Autodesk Inventor part; units mm, degrees
ref_plane "YZ Plane" through (0, 0, 0) normal (1, 0, 0) x (0, 1, 0)
ref_plane "XZ Plane" through (0, 0, 0) normal (0, 1, 0) x (-1, 0, 0)
ref_plane "XY Plane" through (0, 0, 0) normal (0, 0, 1) x (1, 0, 0)
sketch "Sketch1" plane through (0, 0, 0) normal (0, 0, 1) x (1, 0, 0)
  line L0 (0, 0) -> (20, 0)
  line L1 (20, 0) -> (20, 20)
  line L2 (20, 20) -> (0, 20)
  line L3 (0, 20) -> (0, 0)
  dimension "d2" = 20
  dimension "d3" = 20
extrude "Extrusion1" add sketch "Sketch1" along normal blind 5
sketch "Sketch2" plane through (0, 0, 5) normal (0, 0, 1) x (1, 0, 0)
  point P0 (0, 0)
sketch "Sketch3" plane through (0, 0, 5) normal (0, 0, 1) x (1, 0, 0)
  line L0 (0, 0) -> (10, 0)
  line L1 (0, 0) -> (20, 0)
  line L2 (10, 0) -> (10, 10)
  circle A0 centre (10, 10) radius 5
  dimension "d6" = 10
  dimension "d7" = 10
  dimension "d8" = 10
extrude "Extrusion2" add sketch "Sketch3" along normal blind 450
thread "Thread1"
properties part number "bolt for capping system"
The model under review builds one solid part; all positions refer to its coordinate system, in mm. A direction names the side the tool comes from. Round coordinates to 2 decimals unless told otherwise and drop trailing zeros. Loops run counter-clockwise (first coordinate to the right, second up) from the corner with the lowest first, then second, coordinate; pieces in that order, holes last.
1) Clearance check with flat-ended pins moving along their axes: P1, Ø8, axis at x = 18, y = 4, coming from the +Z side; P2, Ø2, axis at y = 8, z = 316.5, coming from the +X side; P3, Ø6, axis at x = 4.5, z = 122.5, coming from the +Y side. State where each tip first meets the part, or that it passes through.
Values follow:
P1: stops at z = 5
P2: stops at x = 14.9
P3: stops at y = 14.33
2) Wall thickness on line 1 along Z through (x, y) = (4.75, 6); line 2 along X through (y, z) = (10.75, 300); line 3 along Y through (x, z) = (10, 292): over which ranges is each line inside the solid? List them lowest first.
Values follow:
line 1: z = 0 to 5
line 2: x = 5.06 to 14.94
line 3: y = 5 to 15
3) Tool access review of faces 1 (the face through (10, 10, 455)), 2 (the face through (8, 15, 5)): name each direction out of +Z, -Z, +X, -X, +Y, -Y from which nothing blocks a thin tool from reaching the whole face with its end or side.
Values follow:
face 1: +Z, +X, -X, +Y, -Y
face 2: +Z
4) Consider section C-C on z = 54. State the section outline as (x, y) points.
Values follow:
outline: circle Ø10 at (10, 10)
5) Consider section A-A on y = 10. State the section outline as (x, z) points, then the cut area to 3 significant figures.
Values follow:
outline: (0, 0) - (20, 0) - (20, 5) - (15, 5) - (15, 455) - (5, 455) - (5, 5) - (0, 5) - close
area: 4,600 mm2
